```python
from build123d import *

# Parameters (mm, degrees)
F0_R     = 5
F3_W     = 26.240948
F3_H     = 20
F4_DEPTH = 12.5
F5_R     = 1.5
F6_DEPTH = 1.4


with BuildPart() as f2:
    # F0 (on Top) → F2 section 0
    with BuildSketch(Plane.XY, mode=Mode.PRIVATE) as f2_s0:
        Circle(F0_R)
    loft([f2_s0.sketch, Vertex(0, 0, 19.961977)])

    # F3 (on Right) → F4 (cut, symmetric)
    with BuildSketch(Plane.YZ):
        with Locations((0, 13.174092)):
            Rectangle(F3_W, F3_H)
    extrude(amount=F4_DEPTH, both=True, mode=Mode.SUBTRACT)

    # F5 (on face) → F6 (cut)
    with BuildSketch(Plane.XY.offset(3.174092)):
        Circle(F5_R)
    extrude(amount=-F6_DEPTH, mode=Mode.SUBTRACT)


solid = f2.part
```
Geometry check sheet. Reference: the model listing, model coordinates, mm. A direction names the side the tool comes from. Give positions to 0.01 mm unless a question says otherwise; leave off trailing zeros. Order: outer loops, then holes, each group sorted by start corner. A loop starts at its lowest first (then second) coordinate and runs counter-clockwise, first axis right, second up.
1. Gauge pin test, flat ends, axial feed: pin 1 Ø1 at (y, z) = (-2, 2.5) entering from -X; pin 2 Ø2 at (x, y) = (-3.5, -3.5) entering from +Z; pin 3 Ø1.5 at (x, z) = (-2.5, 1) entering from +Y; pin 4 Ø2.5 at (x, y) = (0, 0) entering from +Z. Record the tip position at first contact, or that the pin passes through.
2. Section check D-D, the plane z = 2.9. Enter the section's corners in (x, y).
3. Thickness scan on L1, parallel to Z at x = 0.75, y = -0.5; L2, parallel to Y at x = 1.25, z = 2.5; L3, parallel to Y at x = 0, z = 2.6. Record the ranges inside material, lowest first.
4. Section check C-C, the plane z = 1.9. Enter the section's corners in (x, y), and give its area (3 significant figures).
5. Release check for a two-part mould opening along X. For faces 1 (the face through (-0.94, -4.23, 2.67)), 2 (the face through (0, 0, 1.774)), 3 (the face through (0, 0, 0)) record: pulls with the +X half, pulls with the -X half, needs draft (parallel to the pull), parting line crosses it, or undercut.
6. Access from +Z, -Z, +X, -X, +Y, -Y to the whole of each face (thin tool, end or side, straight path). Record for faces 4 (the face through (0, 2, 3.174)), 5 (the face through (-1.5, 0.07, 2.48)).
7. Section check B-B, the plane z = 0.55. Enter the section's corners in (x, y).
8. Section check A-A, the plane x = 0. Enter the section's corners in (y, z).
Values follow:
1. pin 1: stops at x = -4.15
1. pin 2: stops at z = 3.17
1. pin 3: stops at y = 4.48
1. pin 4: stops at z = 1.77
2. outline: circle Ø8.55 at (0, 0); hole circle Ø3 at (0, 0)
3. L1: z = 0 to 1.77
3. L2: y = -4.19 to -0.83, 0.83 to 4.19
3. L3: y = -4.35 to -1.5, 1.5 to 4.35
4. outline: circle Ø9.05 at (0, 0); hole circle Ø3 at (0, 0)
4. area: 57.2 mm2
5. face 1: parting line crosses it
5. face 2: undercut
5. face 3: needs draft
6. face 4: +Z, +X, -X, +Y, -Y
6. face 5: +Z
7. outline: circle Ø9.72 at (0, 0)
8. outline: (-5, 0) - (5, 0) - (4.2, 3.17) - (1.5, 3.17) - (1.5, 1.77) - (-1.5, 1.77) - (-1.5, 3.17) - (-4.2, 3.17) - close
